Can you work these out from the drawing? Everything is in mm from the part's minimum corner. Give positions to 0.01 mm unless a question says otherwise; leave off trailing zeros. Order: outer loops, then holes, each group sorted by start corner. A loop starts at its lowest first (then second) coordinate and runs counter-clockwise, first axis right, second up. Notation, with made-up numbers: (5.25, -34.5) - (19.25, -34.5) arc R22 cw to (19.25, -5.5) - close; hole circle Ø2 at (-39, 64.5). An arc over 180 degrees is marked (long way). One line per question, with ' | ' between items.
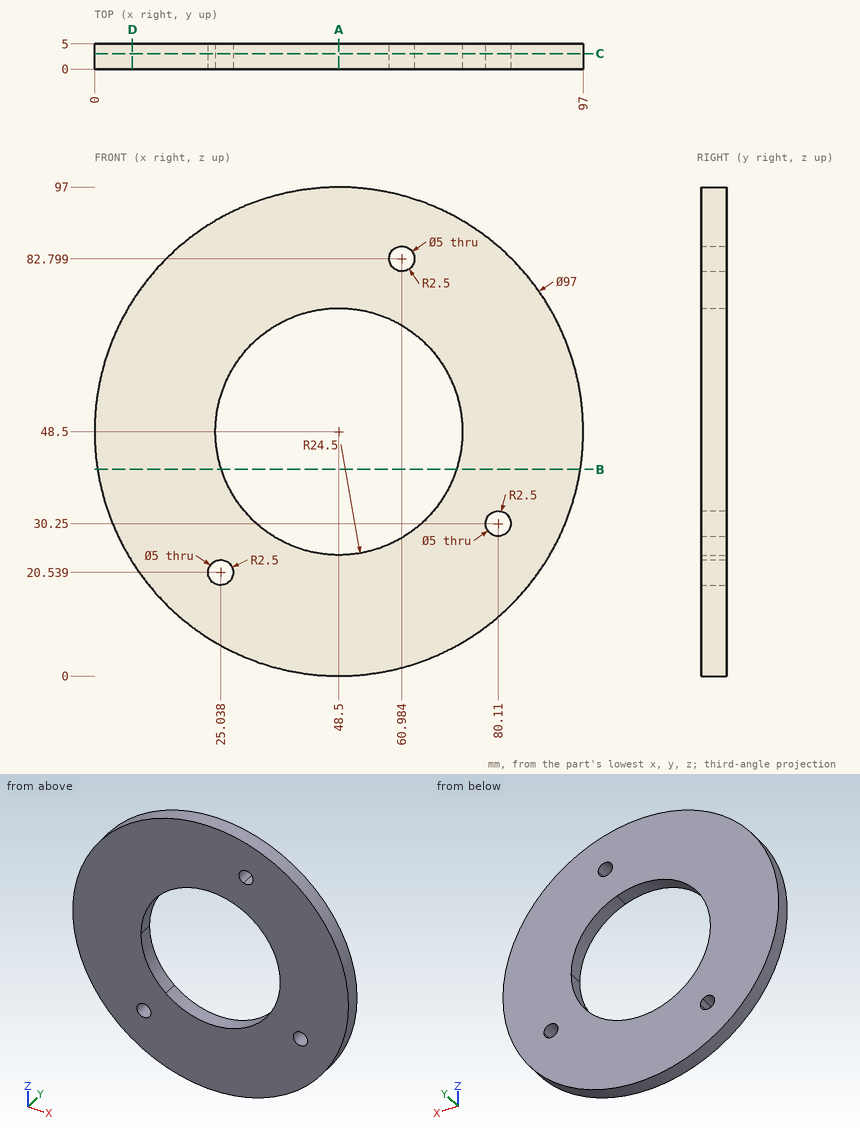
(1) Imagine slicing it at A-A (x = 48.5). List the corners of the cut face in (y, z) for me.
Answer below:
outline: (0, 0) - (5, 0) - (5, 24) - (0, 24) - close; (0, 73) - (5, 73) - (5, 97) - (0, 97) - close
(2) If I drill on line 1 (Z direction, x = 49, y = 3.45) (1 decimal); line 2 (Z direction, x = 59.5, y = 2.3) (1 decimal); line 3 (X direction, y = 1.3, z = 67.5) (1 decimal), over which ranges is the centre line in solid material (lowest first)?
Answer below:
line 1: 0 to 24, 73 to 97 | line 2: 1.3 to 26.6, 70.4 to 80.8, 84.8 to 95.7 | line 3: 3.9 to 33, 64 to 93.1
(3) Will these pins go through, and if not, where does the flat tip stop? pin 1 (2 mm diameter, centred on x = 80, y = 3, fed in from +Z); pin 2 (3 mm diameter, centred on x = 60.98, z = 82.8, fed in from +Y).
Answer below:
pin 1: z = 86.21 | pin 2: through
(4) Imagine slicing it at D-D (x = 7.5). List the corners of the cut face in (y, z) for me.
Answer below:
outline: (0, 22.59) - (5, 22.59) - (5, 74.41) - (0, 74.41) - close
(5) Imagine slicing it at C-C (y = 3.1). Count the separate pieces of the cut face and the enclosed holes in it.
Answer below:
separate pieces: 1 | enclosed holes: 4
(6) Imagine slicing it at B-B (z = 41). List the corners of the cut face in (x, y) for me.
Answer below:
outline: (0.58, 0) - (25.18, 0) - (25.18, 5) - (0.58, 5) - close; (71.82, 0) - (96.42, 0) - (96.42, 5) - (71.82, 5) - close
